```python
from build123d import *

# Parameters (mm, degrees)
SKETCH1_W                  = 31.75
SKETCH1_H                  = 22.098
BOSS_EXTRUDE1_DEPTH        = 12.7
SKETCH2_R                  = 9.525
CUT_EXTRUDE1_DEPTH         = 1.778
F_6_0_204_DIAMETER_HOLE1_D = 5.1816
CUT_EXTRUDE2_REACH         = 14.7
SKETCH5_R                  = 7.62


with BuildPart() as part:
    # Sketch1 → Boss-Extrude1 (new body)
    with BuildSketch(Plane(origin=(0, 0, 0), x_dir=(1, 0, 0), z_dir=(0, 1, 0))):
        Rectangle(SKETCH1_W, SKETCH1_H)
    extrude(amount=BOSS_EXTRUDE1_DEPTH)

    # Sketch2 → Cut-Extrude1 (cut)
    with BuildSketch(Plane(origin=(0, 10.16, 0), x_dir=(1, 0, 0), z_dir=(0, 1, 0))):
        Circle(SKETCH2_R)
    extrude(amount=CUT_EXTRUDE1_DEPTH, mode=Mode.SUBTRACT)

    # #6 (0.204) Diameter Hole1 (through all)
    with Locations(Plane.XY.offset(11.049)):
        with Locations((-9.525, 5.08), (9.525, 5.08)):
            Hole(F_6_0_204_DIAMETER_HOLE1_D / 2)

    # Sketch5 → Cut-Extrude2 (cut, up to next)
    with BuildSketch(Plane(origin=(0, 12.7, 0), x_dir=(1, 0, 0), z_dir=(0, 1, 0)), mode=Mode.PRIVATE) as cut_extrude2_sk1:
        Circle(SKETCH5_R)
    cut_extrude2_tool1 = extrude(cut_extrude2_sk1.sketch, amount=-CUT_EXTRUDE2_REACH, mode=Mode.PRIVATE) & part.part
    add(cut_extrude2_tool1.solids().sort_by_distance((0, 12.7, 0))[0], mode=Mode.SUBTRACT)


solid = part.part
```
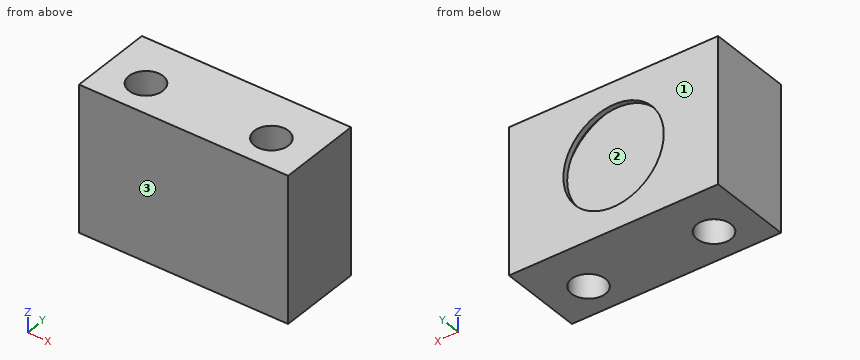
The model under review builds one solid part; all positions refer to its coordinate system, in mm. Face numbers are marked on the shaded views. Round coordinates to 2 decimals unless told otherwise and drop trailing zeros. Loops run counter-clockwise (first coordinate to the right, second up) from the corner with the lowest first, then second, coordinate; pieces in that order, holes last. Notation, with made-up numbers: (54, -2) - (109, -2) arc R16 ccw to (109, 2) - close; hole circle Ø5 at (89.25, 86). An arc over 180 degrees is marked (long way). Use a Markdown table: item, result. Add a question column.
Q1. For probe 1 along X at (y, z) = (12.5, 0) (3 decimals); probe 2 along Z at (x, y) = (0, 12.4); probe 3 along Y at (x, z) = (9.5, 3.75), list the stretches that pass through material, from the lowest coordinate up.
Q2. Add section A-A (y = 5.08). State the section outline as (x, z) points (3 decimals).
Q3. Add section B-B (x = -9). State the section outline as (y, z) points, plus the area to 3 significant figures.
Q4. Add section C-C (z = 0). State the section outline as (x, y) points (3 decimals), plus the area to 3 significant figures.
Q5. The part is to be moulded in two halves that separate along Y. For the marked faces 1, 2 and 3, say which applies: pulls with the +Y half, pulls with the -Y half, needs draft (parallel to the pull), parting line crosses it, or undercut.
Q6. Add section D-D (x = 0). State the section outline as (y, z) points (3 decimals).
Q7. Insertion check: pin 1 Ø9 at (x, z) = (0, 0) entering from -Y; pin 2 Ø4.5 at (x, y) = (9.525, 5.08) entering from -Z. Each pin has a flat end and moves straight along its axis. Give the tip position at first contact, or say it passes through.
Worked answers:
| question | item | result |
|---|---|---|
| 1 | probe 1 | -15.875 to -7.62, 7.62 to 15.875 |
| 1 | probe 2 | -11.05 to -7.62, 7.62 to 11.05 |
| 1 | probe 3 | 0 to 2.49, 7.67 to 12.7 |
| 2 | outline | (-15.875, -11.049) - (-12.116, -11.049) - (-12.116, 11.049) - (-15.875, 11.049) - close; (-6.934, -11.049) - (6.934, -11.049) - (6.934, 11.049) - (-6.934, 11.049) - close; (12.116, -11.049) - (15.875, -11.049) - (15.875, 11.049) - (12.116, 11.049) - close |
| 3 | outline | (0, -11.05) - (2.54, -11.05) - (2.54, 11.05) - (0, 11.05) - close; (7.62, -11.05) - (12.7, -11.05) - (12.7, 11.05) - (7.62, 11.05) - close; hole (10.16, -3.12) - (11.94, -3.12) - (11.94, 3.12) - (10.16, 3.12) - close |
| 3 | area | 157 mm² |
| 4 | outline | (-15.875, 0) - (15.875, 0) - (15.875, 12.7) - (7.62, 12.7) - (7.62, 11.938) - (9.525, 11.938) - (9.525, 10.16) - (-9.525, 10.16) - (-9.525, 11.938) - (-7.62, 11.938) - (-7.62, 12.7) - (-15.875, 12.7) - close; hole circle Ø5.182 at (-9.525, 5.08); hole circle Ø5.182 at (9.525, 5.08) |
| 4 | area | 316 mm² |
| 5 | face 1 | pulls with the +Y half |
| 5 | face 2 | undercut |
| 5 | face 3 | pulls with the -Y half |
| 6 | outline | (0, -11.049) - (12.7, -11.049) - (12.7, -7.62) - (11.938, -7.62) - (11.938, -9.525) - (10.16, -9.525) - (10.16, 9.525) - (11.938, 9.525) - (11.938, 7.62) - (12.7, 7.62) - (12.7, 11.049) - (0, 11.049) - close |
| 7 | pin 1 | y = 0 |
| 7 | pin 2 | through |
